```python
from build123d import *

# Parameters (mm, degrees)
SKETCH2_W           = 63.75
SKETCH2_H           = 7.85
BOSS_EXTRUDE1_DEPTH = 3.15
SKETCH3_R           = 2.45
BOSS_EXTRUDE2_DEPTH = 1.8
SHELL1_T            = -1.5
SKETCH4_R           = 1.5
SKETCH4_R_2         = 0.8
BOSS_EXTRUDE3_DEPTH = 1.45


with BuildPart() as part:
    # Sketch2 → Boss-Extrude1 (new body)
    with BuildSketch(Plane(origin=(0, 0, 0), x_dir=(1, 0, 0), z_dir=(0, 1, 0))):
        Rectangle(SKETCH2_W, SKETCH2_H)
    extrude(amount=-BOSS_EXTRUDE1_DEPTH)

    # Sketch3 → Boss-Extrude2 (add)
    with BuildSketch(Plane(origin=(0, 0, 0), x_dir=(1, 0, 0), z_dir=(0, 1, 0))):
        with Locations(Location((-27.890625, 0, 0), (0, 0, 270))):
            Circle(SKETCH3_R)
        with Locations(Location((-19.921875, 0, 0), (0, 0, 270))):
            Circle(SKETCH3_R)
        with Locations(Location((-11.953125, 0, 0), (0, 0, 270))):
            Circle(SKETCH3_R)
        with Locations(Location((-3.984375, 0, 0), (0, 0, 270))):
            Circle(SKETCH3_R)
        with Locations(Location((3.984375, 0, 0), (0, 0, 270))):
            Circle(SKETCH3_R)
        with Locations(Location((11.953125, 0, 0), (0, 0, 270))):
            Circle(SKETCH3_R)
        with Locations(Location((19.921875, 0, 0), (0, 0, 270))):
            Circle(SKETCH3_R)
        with Locations(Location((27.890625, 0, 0), (0, 0, 270))):
            Circle(SKETCH3_R)
    extrude(amount=BOSS_EXTRUDE2_DEPTH)

    # Shell1
    shell1_openings = [part.faces().sort_by_distance(p)[0] for p in [
        (0, -3.15, 0),
    ]]
    offset(amount=SHELL1_T, openings=shell1_openings, kind=Kind.INTERSECTION)

    # Sketch4 → Boss-Extrude3 (add)
    # profile 1 of 7: a face of its own
    with BuildSketch(Plane.XZ.offset(1.5)):
        with Locations(Location((-23.90625, 0, 0), (0, 0, 90))):
            Circle(SKETCH4_R)
        with Locations(Location((-23.90625, 0, 0), (0, 0, 90))):
            Circle(SKETCH4_R_2, mode=Mode.SUBTRACT)
    # profile 2 of 7: a face of its own
    with BuildSketch(Plane.XZ.offset(1.5)):
        with Locations(Location((-15.9375, 0, 0), (0, 0, 90))):
            Circle(SKETCH4_R)
        with Locations(Location((-15.9375, 0, 0), (0, 0, 90))):
            Circle(SKETCH4_R_2, mode=Mode.SUBTRACT)
    # profile 3 of 7: a face of its own
    with BuildSketch(Plane.XZ.offset(1.5)):
        with Locations(Location((-7.96875, 0, 0), (0, 0, 90))):
            Circle(SKETCH4_R)
        with Locations(Location((-7.96875, 0, 0), (0, 0, 90))):
            Circle(SKETCH4_R_2, mode=Mode.SUBTRACT)
    # profile 4 of 7: a face of its own
    with BuildSketch(Plane.XZ.offset(1.5)):
        with Locations(Location((0, 0, 0), (0, 0, 90))):
            Circle(SKETCH4_R)
        with Locations(Location((0, 0, 0), (0, 0, 90))):
            Circle(SKETCH4_R_2, mode=Mode.SUBTRACT)
    # profile 5 of 7: a face of its own
    with BuildSketch(Plane.XZ.offset(1.5)):
        with Locations(Location((7.96875, 0, 0), (0, 0, 90))):
            Circle(SKETCH4_R)
        with Locations(Location((7.96875, 0, 0), (0, 0, 90))):
            Circle(SKETCH4_R_2, mode=Mode.SUBTRACT)
    # profile 6 of 7: a face of its own
    with BuildSketch(Plane.XZ.offset(1.5)):
        with Locations(Location((15.9375, 0, 0), (0, 0, 90))):
            Circle(SKETCH4_R)
        with Locations(Location((15.9375, 0, 0), (0, 0, 90))):
            Circle(SKETCH4_R_2, mode=Mode.SUBTRACT)
    # profile 7 of 7: a face of its own
    with BuildSketch(Plane.XZ.offset(1.5)):
        with Locations(Location((23.90625, 0, 0), (0, 0, 90))):
            Circle(SKETCH4_R)
        with Locations(Location((23.90625, 0, 0), (0, 0, 90))):
            Circle(SKETCH4_R_2, mode=Mode.SUBTRACT)
    extrude(amount=BOSS_EXTRUDE3_DEPTH)


solid = part.part
```
The model under review builds one solid part; all positions refer to its coordinate system, in mm. A direction names the side the tool comes from. Round coordinates to 2 decimals unless told otherwise and drop trailing zeros. Loops run counter-clockwise (first coordinate to the right, second up) from the corner with the lowest first, then second, coordinate; pieces in that order, holes last. Notation, with made-up numbers: (-34.75, 68.5) - (-28.75, 68.5) arc R15 ccw to (-28.75, 74.5) - close; hole circle Ø2 at (14, -1). An arc over 180 degrees is marked (long way). Use a Markdown table: item, result. Add a question column.
Q1. Add section A-A (y = -2.4). State how many separate pieces and enclosed holes the cut face has, plus the area to 3 significant figures.
Q2. Insertion check: pin 1 Ø3 at (x, z) = (-19, 1) entering from -Y; pin 2 Ø0.9 at (x, z) = (8, 0) entering from -Y; pin 3 Ø1.1 at (x, z) = (19.92, 0) entering from -Y; pin 4 Ø3 at (x, z) = (-0.5, 2) entering from +Y. Each pin has a flat end and moves straight along its axis. Give the tip position at first contact, or say it passes through.
Q3. For probe 1 along Z at (x, y) = (8, -1.7) (3 decimals); probe 2 along Z at (x, y) = (2.5, -2.8) (3 decimals); probe 3 along Y at (x, z) = (28, 2.25), list the stretches that pass through material, from the lowest coordinate up.
Q4. Machinability: for faces 5 (the face through (12, 1.8, 0)), 6 (the face through (0, 0, 0)), 7 (the face through (0, -2, 2.425)), which of the approach directions +Z, -Z, +X, -X, +Y, -Y give a long, thin tool a straight path to every point of the face, cutting with its end or side? Answer none if there is none.
Q5. Add section D-D (x = 21.5). State the section outline as (y, z) points (3 decimals).
Q6. Add section C-C (x = 0). State the section outline as (y, z) points (3 decimals), plus the area to 3 significant figures.
Q7. The part is to be moulded in two halves that separate along Z. For faces 1 (the face through (-28, 1.8, 0)), 2 (the face through (6.414, 0.887, -0.319)), 3 (the face through (-28, 0.3, 0)), 4 (the face through (0.49, -2.21, -0.63)), say which applies: pulls with the +Z half, pulls with the -Z half, needs draft (parallel to the pull), parting line crosses it, or undercut.
Q8. Add section B-B (y = 1.15). State the section outline as (x, z) points.
Worked answers:
| question | item | result |
|---|---|---|
| 1 | separate pieces | 8 |
| 1 | enclosed holes | 8 |
| 1 | area | 241 mm² |
| 2 | pin 1 | y = -3.15 |
| 2 | pin 2 | y = -1.5 |
| 2 | pin 3 | y = 0.3 |
| 2 | pin 4 | y = 0 |
| 3 | probe 1 | -3.925 to -2.425, -1.5 to -0.799, 0.799 to 1.5, 2.425 to 3.925 |
| 3 | probe 2 | -3.925 to -2.425, 2.425 to 3.925 |
| 3 | probe 3 | -1.5 to 1.8 |
| 4 | face 5 | +Z, -Z, +X, -X, +Y |
| 4 | face 6 | +Y |
| 4 | face 7 | -Y |
| 5 | outline | (-3.15, -3.925) - (0, -3.925) - (0, -1.874) - (1.8, -1.874) - (1.8, 1.874) - (0, 1.874) - (0, 3.925) - (-3.15, 3.925) - (-3.15, 2.425) - (-1.5, 2.425) - (-1.5, -2.425) - (-3.15, -2.425) - close |
| 6 | outline | (-3.15, -3.925) - (0, -3.925) - (0, 3.925) - (-3.15, 3.925) - (-3.15, 2.425) - (-1.5, 2.425) - (-1.5, 1.5) - (-2.95, 1.5) - (-2.95, 0.8) - (-1.5, 0.8) - (-1.5, -0.8) - (-2.95, -0.8) - (-2.95, -1.5) - (-1.5, -1.5) - (-1.5, -2.425) - (-3.15, -2.425) - close |
| 6 | area | 18.8 mm² |
| 7 | face 1 | needs draft |
| 7 | face 2 | parting line crosses it |
| 7 | face 3 | undercut |
| 7 | face 4 | undercut |
| 8 | outline | circle Ø4.9 at (-27.89, 0); circle Ø4.9 at (-19.92, 0); circle Ø4.9 at (-11.95, 0); circle Ø4.9 at (-3.98, 0); circle Ø4.9 at (3.98, 0); circle Ø4.9 at (11.95, 0); circle Ø4.9 at (19.92, 0); circle Ø4.9 at (27.89, 0) |
